```python
from build123d import *

# Parameters (mm, degrees)
SKETCH1_R           = 9
BOSS_EXTRUDE1_DEPTH = 6
SKETCH2_R           = 12
CUT_EXTRUDE1_DEPTH  = 5
SKETCH3_R           = 2
CUT_EXTRUDE2_DEPTH  = 10
FILLET1_R           = 3


with BuildPart() as part:
    # Sketch1 → Boss-Extrude1 (new body, symmetric)
    with BuildSketch(Plane.XY):
        with BuildLine():
            Line((-35, 21), (35, 21))
            Line((35, 21), (35, 0))
            Line((35, 0), (31.622776602, 0))
            ThreePointArc((31.622776602, 0), (23.604939344, -2.322686179), (18.070158058, -8.571428571))
            ThreePointArc((18.070158058, -8.571428571), (0, -20), (-18.070158058, -8.571428571))
            ThreePointArc((-18.070158058, -8.571428571), (-23.604939344, -2.322686179), (-31.622776602, 0))
            Line((-31.622776602, 0), (-35, 0))
            Line((-35, 0), (-35, 21))
        make_face()
        Circle(SKETCH1_R, mode=Mode.SUBTRACT)
    extrude(amount=BOSS_EXTRUDE1_DEPTH, both=True)

    # Sketch2 → Cut-Extrude1 (cut)
    with BuildSketch(Plane(origin=(0, 0, -6), x_dir=(-1, 0, 0), z_dir=(0, 0, -1))):
        Circle(SKETCH2_R)
    extrude(amount=-CUT_EXTRUDE1_DEPTH, mode=Mode.SUBTRACT)

    # Sketch3 → Cut-Extrude2 (cut)
    with BuildSketch(Plane(origin=(0, 21, 0), x_dir=(1, 0, 0), z_dir=(0, 1, 0))):
        with Locations((-29, 0)):
            Circle(SKETCH3_R)
        with Locations((29, 0)):
            Circle(SKETCH3_R)
    extrude(amount=-CUT_EXTRUDE2_DEPTH, mode=Mode.SUBTRACT)

    # Fillet1
    fillet1_edges = [part.edges().sort_by_distance(p)[0] for p in [
        (0, -20, -6),
        (-23.604939344, -2.322686179, -6),
        (-33.311388301, 0, -6),
        (33.311388301, 0, -6),
        (23.604939344, -2.322686179, -6),
    ]]
    fillet(fillet1_edges, radius=FILLET1_R)


solid = part.part
```
Check sheet for the modelled part. Datum: model origin and axes. Units: mm. A direction names the side the tool comes from. Round coordinates to 2 decimals unless told otherwise and drop trailing zeros. Loops run counter-clockwise (first coordinate to the right, second up) from the corner with the lowest first, then second, coordinate; pieces in that order, holes last. Notation, with made-up numbers: (18, 4) -> (22, 4) arc R13 ccw to (22, 9) -> close; hole circle Ø1 at (23.5, 88.25). An arc over 180 degrees is marked (long way). Write item = value, one per line. Start each with the question number.
1) Sectioned sample at A-A, the plane x = 0. Record the cut outline in (y, z).
2) Sectioned sample at B-B, the plane z = 5. Record the cut outline in (x, y), plus the area to 3 significant figures.
3) Thickness scan on probe 1 along X at (y, z) = (16, 0); probe 2 along Z at (x, y) = (29, 18); probe 3 along Y at (x, z) = (0, 3.5). Record the ranges inside material, lowest first.
4) Sectioned sample at C-C, the plane y = 5. Record the cut outline in (x, z), plus the area to 3 significant figures.
5) Set-up check for faces 4 (the cylindrical face through (11.99, 0.53, -3.54)), 5 (the flat face through (-29, 11, 0)), 6 (the cylindrical face through (33.29, 0.9, -5.14)), 7 (the cylindrical face through (-33.34, 0.9, -5.14)), 8 (the flat face through (-33, 0, 2)): record each of +Z, -Z, +X, -X, +Y, -Y from which the full face is reachable in a straight line by a thin tool's end or side.
6) Sectioned sample at D-D, the plane y = 17. Record the cut outline in (x, z).
7) Gauge pin test, flat ends, axial feed: pin 1 Ø14.5 at (x, y) = (0, 0) entering from +Z; pin 2 Ø2.5 at (x, z) = (-34, 2.5) entering from -Y; pin 3 Ø5 at (x, z) = (29, 0) entering from -Y; pin 4 Ø1.2 at (x, z) = (28.5, 0.5) entering from +Y. Record the tip position at first contact, or that the pin passes through.
8) Release check for a two-part mould opening along Z. For faces 1 (the cylindrical face through (-27.092, 16.07, -0.601)), 2 (the flat face through (0, 10, 6)), 3 (the flat face through (33, 0, 2)) record: released by +Z, released by -Z, zero draft, split by the parting line, or undercut.
Results are:
q1.outline = (-20, -3) arc R3 ccw to (-17, -6) -> (-12, -6) -> (-12, -1) -> (-9, -1) -> (-9, 6) -> (-20, 6) -> close; (9, -1) -> (12, -1) -> (12, -6) -> (21, -6) -> (21, 6) -> (9, 6) -> close
q2.outline = (-35, 0) -> (-31.62, 0) arc R15 cw to (-18.07, -8.57) arc R20 ccw to (18.07, -8.57) arc R15 cw to (31.62, 0) -> (35, 0) -> (35, 21) -> (-35, 21) -> close; hole circle Ø18 at (0, 0)
q2.area = 1,890 mm^2
q3.probe_1 = -35 to -31, -27 to 27, 31 to 35
q3.probe_2 = -6 to -2, 2 to 6
q3.probe_3 = -20 to -9, 9 to 21
q4.outline = (-35, -6) -> (-10.91, -6) -> (-10.91, -1) -> (-7.48, -1) -> (-7.48, 6) -> (-35, 6) -> close; (7.48, -1) -> (10.91, -1) -> (10.91, -6) -> (35, -6) -> (35, 6) -> (7.48, 6) -> close
q4.area = 626 mm^2
q5.face_4 = -Z
q5.face_5 = +Y
q5.face_6 = -Z, +X, -Y
q5.face_7 = -Z, -X, -Y
q5.face_8 = +Z, -Z, -X, -Y
q6.outline = (-35, -6) -> (35, -6) -> (35, 6) -> (-35, 6) -> close; hole circle Ø4 at (-29, 0); hole circle Ø4 at (29, 0)
q7.pin_1 = through
q7.pin_2 = 0
q7.pin_3 = -0.9
q7.pin_4 = 11
q8.face_1 = undercut
q8.face_2 = released by +Z
q8.face_3 = zero draft
